from build123d import *

# Parameters (mm, degrees)
SKETCH1_R           = 35
BOSS_EXTRUDE1_DEPTH = 3.175
CUT_EXTRUDE1_REACH  = 5.175


with BuildPart() as part:
    # Sketch1 → Boss-Extrude1 (new body)
    with BuildSketch(Plane.XY):
        Circle(SKETCH1_R)
    extrude(amount=BOSS_EXTRUDE1_DEPTH)

    # Sketch2 → Cut-Extrude1 (cut, up to next)
    with BuildSketch(Plane.XY.offset(3.175), mode=Mode.PRIVATE) as cut_extrude1_sk1:
        Polygon((7.505553499, 0), (3.75277675, 6.5), (-3.75277675, 6.5), (-7.505553499, 0), (-3.75277675, -6.5), (3.75277675, -6.5), align=None)
    cut_extrude1_tool1 = extrude(cut_extrude1_sk1.sketch, amount=-CUT_EXTRUDE1_REACH, mode=Mode.PRIVATE) & part.part
    add(cut_extrude1_tool1.solids().sort_by_distance((0, 0, 3.175))[0], mode=Mode.SUBTRACT)


solid = part.part
Can you work these out from the model? Positions are in its coordinate system, mm. A direction names the side the tool comes from. Give positions to 0.01 mm unless a question says otherwise; leave off trailing zeros. Loops run counter-clockwise (first coordinate to the right, second up) from the corner with the lowest first, then second, coordinate; pieces in that order, holes last. Notation, with made-up numbers: M 88,88 L 146,88 A19 ccw 146,115 Z; hole C 61.5,40 d1. An arc over 180 degrees is marked long. One line per item, written item: value. Start each with the question number.
1) If we section it at C-C, the plane y = 1: Write out the boundary of the cut face in (x, z) (3 decimals), and give its area (3 significant figures).
2) If we section it at B-B, the plane z = 1.9: Write out the boundary of the cut face in (x, y), and give its area (3 significant figures).
3) Thinking about a two-plate mould opening in X: for faces 1 (the face through (0, -6.5, 2)), 2 (the face through (0, -7, 0)), 3 (the face through (-28, -21, 2)), which applies, +X half, -X half, draft (parallel to the pull), parting line (faces both ways), or undercut?
4) If we section it at A-A, the plane x = 0: Write out the boundary of the cut face in (y, z) (3 decimals).
5) I'm going to push flat-ended pins straight in: pin 1 (1 mm diameter, centred on x = -22.5, z = 2, fed in from +Y); pin 2 (1 mm diameter, centred on x = 1, z = 1.5, fed in from +Y); pin 3 (1 mm diameter, centred on y = 6.5, z = 2.5, fed in from -X). Where does each tip first touch, or does it pass through?
6) If we section it at D-D, the plane y = 25.5: Write out the boundary of the cut face in (x, z) (3 decimals).
7) If I drill on line 1 (X direction, y = -2, z = 0.8); line 2 (X direction, y = -6, z = 2.85); line 3 (Y direction, x = -6.5, z = 0.8), over which ranges is the centre line in solid material (lowest first)? Write a range as [from, to].
8) On a 3-axis mill with a long thin cutter (end or side, diameter ignored), from which of +Z, -Z, +X, -X, +Y, -Y can I reach the whole of each face in a straight line? I mean faces 4 (the face through (0, -7, 3.175)), 5 (the face through (-5.66, -3.2, 1.61)). Say none if no direction works.
Completed:
1. outline: M -34.986,0 L -6.928,0 L -6.928,3.175 L -34.986,3.175 Z; M 6.928,0 L 34.986,0 L 34.986,3.175 L 6.928,3.175 Z
1. area: 178 mm^2
2. outline: C 0,0 d70; hole M -7.51,0 L -3.75,-6.5 L 3.75,-6.5 L 7.51,0 L 3.75,6.5 L -3.75,6.5 Z
2. area: 3,700 mm^2
3. face 1: undercut
3. face 2: draft
3. face 3: parting line
4. outline: M -35,0 L -6.5,0 L -6.5,3.175 L -35,3.175 Z; M 6.5,0 L 35,0 L 35,3.175 L 6.5,3.175 Z
5. pin 1: stops at y = 27.22
5. pin 2: stops at y = 35
5. pin 3: stops at x = -34.48
6. outline: M -23.974,0 L 23.974,0 L 23.974,3.175 L -23.974,3.175 Z
7. line 1: x = [-34.94, -6.35], [6.35, 34.94]
7. line 2: x = [-34.48, -4.04], [4.04, 34.48]
7. line 3: y = [-34.39, -1.74], [1.74, 34.39]
8. face 4: +Z, +X, -X, +Y, -Y
8. face 5: +Z, -Z
